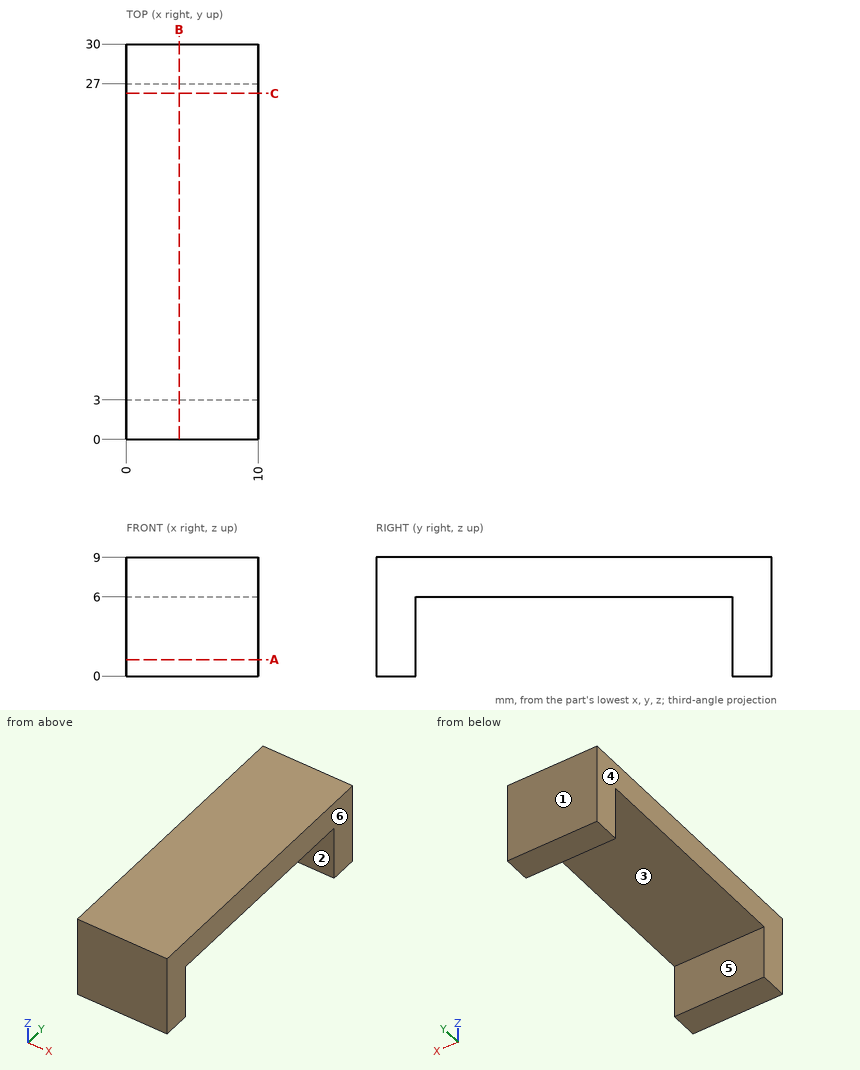
Geometry: see drawing. Coordinates: mm, zero at the bounding-box minimum. A direction names the side the tool comes from. Coordinates: 2 decimals unless noted, no trailing zeros. Loops run counter-clockwise (first coordinate to the right, second up) from the corner with the lowest first, then second, coordinate; pieces in that order, holes last. Notation, with made-up numbers: (-3, -17.5) - (51, -17.5) arc R18 ccw to (51, -2.5) - close; hole circle Ø7 at (26, 62.25). An arc over 180 degrees is marked (long way). Return JSON: item names as keys, results as strings.
Q1. Section B-B, the plane x = 4. Return loops of the section in (y, z), plus the area to 3 significant figures.
Results:
{"outline": "(0, 0) - (3, 0) - (3, 6) - (27, 6) - (27, 0) - (30, 0) - (30, 9) - (0, 9) - close", "area": "126 mm2"}
Q2. Access query for the marked faces 5 and 6. Directions: +Z, -Z, +X, -X, +Y, -Y. A direction counts if a zero-diameter tool reaches every point of the face in a straight line with its end or side. Return the directions, or none.
Results:
{"face 5": "-Z, +X, -X", "face 6": "+Z, -Z, +X, +Y, -Y"}
Q3. Material intervals for line 1 along Y through (x, z) = (1, 5); line 2 along Z through (x, y) = (4.75, 9), sorted ascending.
Results:
{"line 1": "0 to 3, 27 to 30", "line 2": "6 to 9"}
Q4. Section C-C, the plane y = 26.25. Return loops of the section in (x, z), plus the area to 3 significant figures.
Results:
{"outline": "(0, 6) - (10, 6) - (10, 9) - (0, 9) - close", "area": "30.0 mm2"}
Q5. Section A-A, the plane z = 1.25. Return loops of the section in (x, y).
Results:
{"outline": "(0, 0) - (10, 0) - (10, 3) - (0, 3) - close; (0, 27) - (10, 27) - (10, 30) - (0, 30) - close"}
Q6. Mould query, pull axis Y, two halves, no side actions, for the marked faces 1, 2, 3 and 4. Classes: released by +Y, released by -Y, zero draft, split by the parting line, or undercut.
Results:
{"face 1": "released by +Y", "face 2": "undercut", "face 3": "undercut", "face 4": "zero draft"}
Q7. Contact query for flat-ended pins moving along their axis: P1, Ø5, axis at x = 8.5, y = 27, coming from the -Z side; P2, Ø1, axis at x = 7.5, y = 10, coming from the -Z side. Output: stop coordinate, or through.
Results:
{"P1": "z = 0", "P2": "z = 6"}
